For this review, take the finished solid that the model builds, in its own axes (mm). A direction names the side the tool comes from. Give positions to 0.01 mm unless a question says otherwise; leave off trailing zeros. Loops run counter-clockwise (first coordinate to the right, second up) from the corner with the lowest first, then second, coordinate; pieces in that order, holes last. Notation, with made-up numbers: (50.5, -12.75) - (104.5, -12.75) arc R10 cw to (104.5, -3.75) - close; hole circle Ø3 at (-20, -20.5). An arc over 180 degrees is marked (long way). Answer in a Markdown table with one row per item.
```python
from build123d import *

# Parameters (mm, degrees)
SKETCH1_R               = 4.15
BOSS_EXTRUDE1_DEPTH     = 4.8
SKETCH2_R               = 2.5
BOSS_EXTRUDE2_DEPTH     = 20
CUT_EXTRUDE1_DEPTH      = 26.484995586
CUT_EXTRUDE1_DEPTH_BACK = 2.5
CHAMFER1_SIZE           = 0.7
FILLET1_R               = 0.4


with BuildPart() as part:
    # Sketch1 → Boss-Extrude1 (new body)
    with BuildSketch(Plane(origin=(0, 0, 0), x_dir=(1, 0, 0), z_dir=(0, 1, 0))):
        with Locations(Location((0, 0, 0), (0, 0, 270))):
            Circle(SKETCH1_R)
    extrude(amount=BOSS_EXTRUDE1_DEPTH)

    # Sketch2 → Boss-Extrude2 (add)
    with BuildSketch(Plane(origin=(0, 4.8, 0), x_dir=(1, 0, 0), z_dir=(0, 1, 0))):
        with Locations(Location((0, 0, 0), (0, 0, 270))):
            Circle(SKETCH2_R)
    extrude(amount=BOSS_EXTRUDE2_DEPTH)

    # Sketch3 → Cut-Extrude1 (cut, two sides: drawn at the far end of the back side and taken through both)
    with BuildSketch(Plane.XZ.offset(-CUT_EXTRUDE1_DEPTH_BACK)):
        Polygon((2.886751346, 0), (1.443375673, 2.5), (-1.443375673, 2.5), (-2.886751346, 0), (-1.443375673, -2.5), (1.443375673, -2.5), align=None)
    extrude(amount=CUT_EXTRUDE1_DEPTH + CUT_EXTRUDE1_DEPTH_BACK, mode=Mode.SUBTRACT)

    # Chamfer1
    chamfer1_edges = [part.edges().sort_by_distance(p)[0] for p in [
        (0, 24.8, -2.5),
    ]]
    chamfer(chamfer1_edges, length=CHAMFER1_SIZE)

    # Fillet1
    fillet1_edges = [part.edges().sort_by_distance(p)[0] for p in [
        (0, 0, -4.15),
        (0, 4.8, -4.15),
    ]]
    fillet(fillet1_edges, radius=FILLET1_R)


solid = part.part
```
1. Clearance check with flat-ended pins moving along their axes: pin 1 (2 mm diameter, centred on x = 1, y = 17.5, fed in from +Z); pin 2 (1 mm diameter, centred on y = 18.5, z = 1, fed in from +X); pin 3 (3 mm diameter, centred on y = 15, z = 1, fed in from +X). State where each tip first meets the part, or that it passes through.
Values:
| item | result |
|---|---|
| pin 1 | stops at z = 2.5 |
| pin 2 | stops at x = 2.45 |
| pin 3 | stops at x = 2.5 |
2. Mouldability with a two-part tool opening along X and no side actions: class faces 1 (the face through (-2.53, 2.37, -3.29)), 2 (the face through (-2.175, 1.268, -1.233)), 3 (the face through (0, 1, -2.5)), 4 (the face through (3, 4.8, 0)) as released by +X, released by -X, zero draft, split by the parting line, or undercut.
Values:
| item | result |
|---|---|
| face 1 | split by the parting line |
| face 2 | undercut |
| face 3 | undercut |
| face 4 | zero draft |
3. Wall thickness on line 1 (Y direction, x = 1.5, z = 1); line 2 (X direction, y = 1, z = 2); line 3 (Y direction, x = -3.5, z = -0.75): over which ranges is each line inside the solid? List them lowest first. Write a range as [from, to].
Values:
| item | result |
|---|---|
| line 1 | y = [2.5, 24.8] |
| line 2 | x = [-3.64, -1.73], [1.73, 3.64] |
| line 3 | y = [0, 4.8] |
4. We need section A-A, the plane x = 0. Give the boundary of the cut face in (y, z), and give its area (3 significant figures).
Values:
| item | result |
|---|---|
| outline | (0, -3.75) arc R0.4 ccw to (0.4, -4.15) - (4.4, -4.15) arc R0.4 ccw to (4.8, -3.75) - (4.8, -2.5) - (24.1, -2.5) - (24.8, -1.8) - (24.8, 1.8) - (24.1, 2.5) - (4.8, 2.5) - (4.8, 3.75) arc R0.4 ccw to (4.4, 4.15) - (0.4, 4.15) arc R0.4 ccw to (0, 3.75) - (0, 2.5) - (2.5, 2.5) - (2.5, -2.5) - (0, -2.5) - close |
| area | 127 mm^2 |
5. We need section B-B, the plane y = 10. Give the boundary of the cut face in (x, z), and give its area (3 significant figures).
Values:
| item | result |
|---|---|
| outline | circle Ø5 at (0, 0) |
| area | 19.6 mm^2 |
6. For faces 5 (the face through (-2.44, 14.31, -0.54)), 6 (the face through (0, 0, -3)), 7 (the face through (2.155, 1.268, -1.267)), list the 3-axis set-ups (+Z, -Z, +X, -X, +Y, -Y) from which the entire face can be reached by the end or side of a thin tool; tool diameter is ignored.
Values:
| item | result |
|---|---|
| face 5 | +Y |
| face 6 | +Z, -Z, +X, -X, -Y |
| face 7 | -Y |
